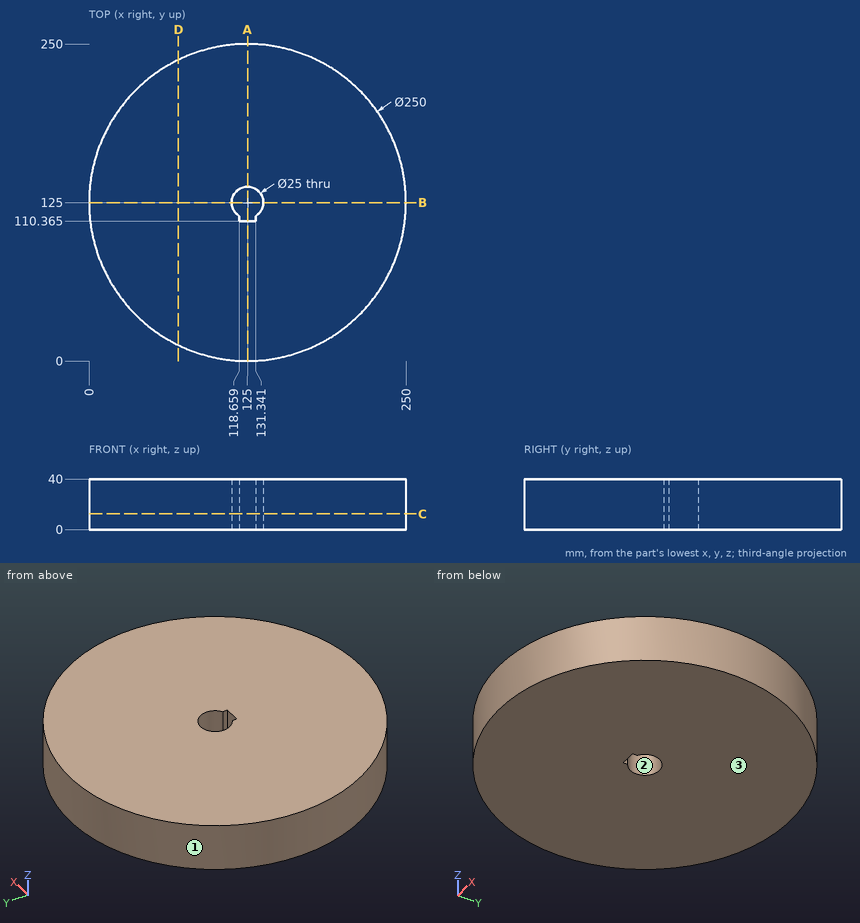
Input: dimensioned drawing with shaded views. Units: mm. Origin: part minimum x, y, z. Give positions to 0.01 mm unless a question says otherwise; leave off trailing zeros. Write each loop counter-clockwise with the first axis right and the second up, starting at its lowest first coordinate (ties: lowest second). Pieces come first, ordered by that corner, then holes.
Q1. Section C-C, the plane z = 12.5. Output: boundary loops of the cut face in (x, y) (1 decimal), plus the area to 3 significant figures.
Q2. Section B-B, the plane y = 125. Output: boundary loops of the cut face in (x, z), plus the area to 3 significant figures.
Q3. Section D-D, the plane x = 70.5. Output: boundary loops of the cut face in (y, z).
Q4. Pull-direction query (X, two-part tool) for the marked faces 1, 2 and 3; classes: pulls with the +X half, pulls with the -X half, needs draft (parallel to the pull), parting line crosses it, or undercut.
Q5. First-contact query: P1, Ø6, axis at x = 212.5, z = 25, coming from the -Y side; P2, Ø1.9, axis at y = 113, z = 28, coming from the +X side; P3, Ø1.5, axis at y = 181, z = 26, coming from the -X side; P4, Ø22.5, axis at x = 125, y = 125, coming from the +Z side. Flat tips, straight axial feed; report the tip coordinate or a pass-through.
Q6. Section A-A, the plane x = 125. Output: boundary loops of the cut face in (y, z) (1 decimal).
Q7. Material intervals for probe 1 along Y at (x, z) = (121, 19) (1 decimal); probe 2 along X at (y, z) = (29.5, 27.5); probe 3 along Y at (x, z) = (183.5, 34.5) (1 decimal), sorted ascending.
Filled in:
1. outline: circle Ø250 at (125, 125); hole (118.7, 110.4) - (131.3, 110.4) - (131.3, 114.2) arc R12.5 ccw (long way) to (118.7, 114.2) - close
1. area: 48,600 mm2
2. outline: (0, 0) - (112.5, 0) - (112.5, 40) - (0, 40) - close; (137.5, 0) - (250, 0) - (250, 40) - (137.5, 40) - close
2. area: 9,000 mm2
3. outline: (12.51, 0) - (237.49, 0) - (237.49, 40) - (12.51, 40) - close
4. face 1: parting line crosses it
4. face 2: undercut
4. face 3: needs draft
5. P1: stops at y = 32.89
5. P2: stops at x = 249.51
5. P3: stops at x = 12.87
5. P4: passes through
6. outline: (0, 0) - (110.4, 0) - (110.4, 40) - (0, 40) - close; (137.5, 0) - (250, 0) - (250, 40) - (137.5, 40) - close
7. probe 1: y = 0.1 to 110.4, 136.8 to 249.9
7. probe 2: x = 44.35 to 205.65
7. probe 3: y = 14.5 to 235.5
